Can you work these out from the drawing? Everything is in mm from the part's minimum corner. Give positions to 0.01 mm unless a question says otherwise; leave off trailing zeros. Loops run counter-clockwise (first coordinate to the right, second up) from the corner with the lowest first, then second, coordinate; pieces in that order, holes last. Notation, with made-up numbers: (-0.75, -36.75) - (9.25, -36.75) arc R27 ccw to (9.25, -3.75) - close; hole circle Ø5 at (18.5, 55). An arc over 180 degrees is marked (long way). Write each question's results on one line, items separated by ' | '. Start each with the question number.
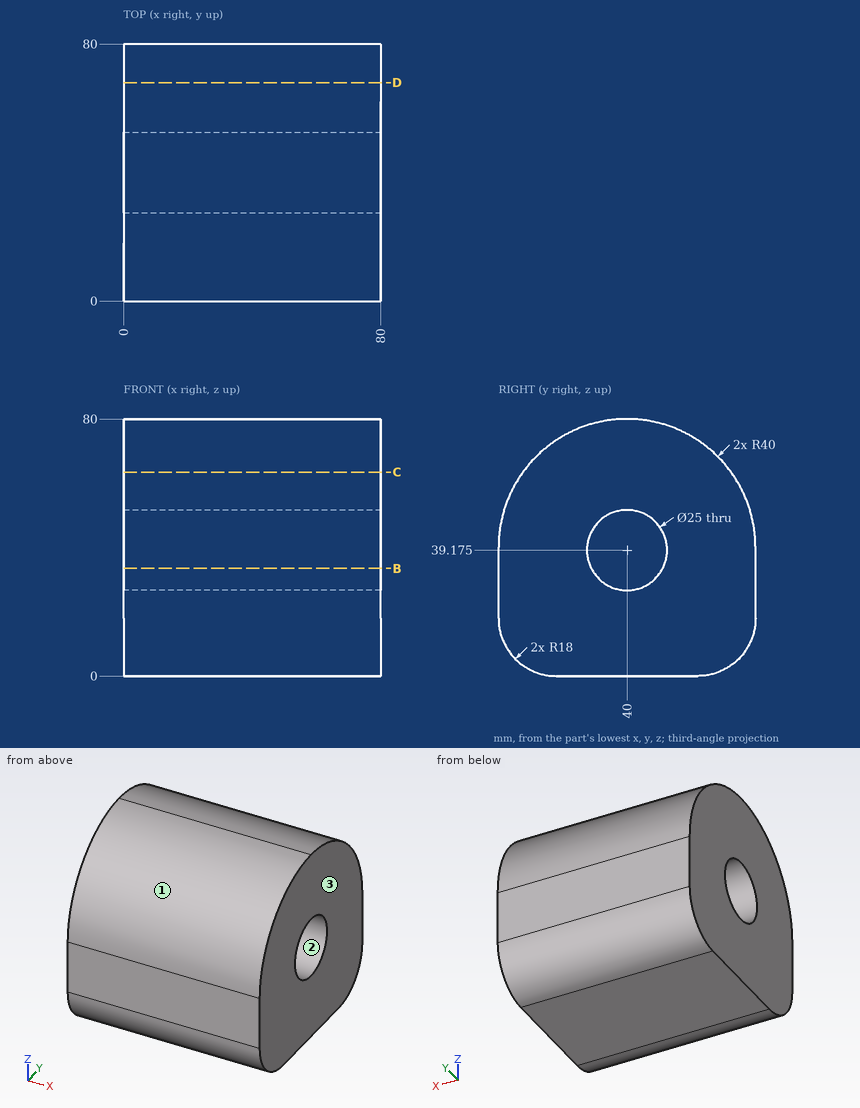
Q1. I need wall thicknesses on L1, parallel to Y at x = 13, z = 49.5 (1 decimal); L2, parallel to Z at x = 50, y = 51.5 (1 decimal); L3, parallel to Y at x = 5, z = 28.5 (1 decimal). Which ranges of each line are inside material? Lowest first, please. Write a range as from..to.
Q2. I'm going to push flat-ended pins straight in: pin 1 Ø10 at (x, z) = (32, 59.5) entering from -Y; pin 2 Ø5 at (x, z) = (19.5, 55.5) entering from -Y; pin 3 Ø4 at (x, y) = (43, 10) entering from +Z (1 decimal). Where does each tip first touch, or does it pass through?
Q3. I want a section at B-B, the plane z = 33.5. List the corners of the cut face in (x, y) for me, then the cut area to 3 significant figures.
Q4. I want a section at D-D, the plane y = 68. List the corners of the cut face in (x, z) for me.
Q5. I want a section at C-C, the plane z = 63.5. List the corners of the cut face in (x, y) for me.
Q6. If we mould it in two halves opening along Z, with no side actions, what happens to the marked faces 1, 2 and 3? For each: +Z half, -Z half, draft (parallel to the pull), parting line (faces both ways), or undercut.
Conclusion:
1) L1: 1.1..33, 47..78.9 | L2: 0..34.3, 44.1..78.3 | L3: 0..33.5, 46.5..80
2) pin 1: y = 2.72 | pin 2: y = 2.17 | pin 3: z = 68.6
3) outline: (0, 0) - (80, 0) - (80, 28.86) - (0, 28.86) - close; (0, 51.14) - (80, 51.14) - (80, 80) - (0, 80) - close | area: 4,620 mm^2
4) outline: (0, 1.03) - (80, 1.03) - (80, 68.57) - (0, 68.57) - close
5) outline: (0, 7.63) - (80, 7.63) - (80, 72.37) - (0, 72.37) - close
6) face 1: +Z half | face 2: undercut | face 3: draft
